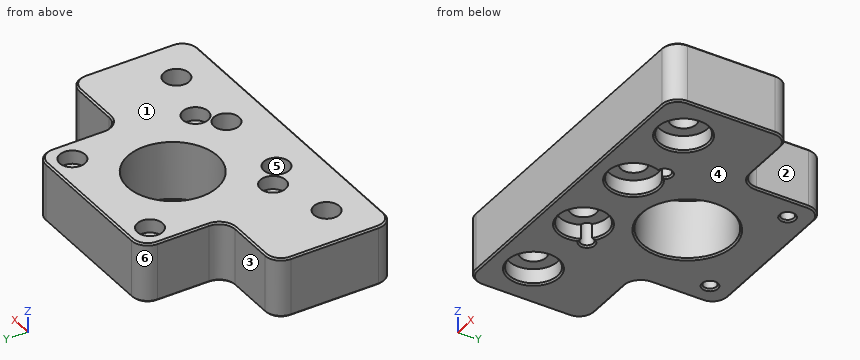
```python
from build123d import *

# Parameters (mm, degrees)
SKETCH_R        = 11.3
SKETCH_R_2      = 1.6
SKETCH_R_3      = 3.2
PAD_DEPTH       = 15
SKETCH001_R     = 3.2
POCKET_DEPTH    = 3.4
SKETCH002_R     = 6.1
POCKET001_DEPTH = 4
FILLET_R        = 4
CHAMFER_SIZE    = 0.4
CHAMFER001_SIZE = 0.4


with BuildPart() as part:
    # Sketch → Pad (new body)
    with BuildSketch(Plane.XY):
        Polygon((20, 30), (20, 51), (62.3, 51), (62.3, 30), (82.3, 30), (82.3, 0), (0, 0), (0, 30), align=None)
        with Locations((41.15, 29.85)):
            Circle(SKETCH_R, mode=Mode.SUBTRACT)
        with Locations((25.65, 45.35)):
            Circle(SKETCH_R_2, mode=Mode.SUBTRACT)
        with Locations((25.65, 14.35)):
            Circle(SKETCH_R_2, mode=Mode.SUBTRACT)
        with Locations((56.65, 45.35)):
            Circle(SKETCH_R_2, mode=Mode.SUBTRACT)
        with Locations((56.65, 14.35)):
            Circle(SKETCH_R_2, mode=Mode.SUBTRACT)
        with Locations((11.15, 10)):
            Circle(SKETCH_R_3, mode=Mode.SUBTRACT)
        with Locations((31.15, 10)):
            Circle(SKETCH_R_3, mode=Mode.SUBTRACT)
        with Locations((51.15, 10)):
            Circle(SKETCH_R_3, mode=Mode.SUBTRACT)
        with Locations((71.15, 10)):
            Circle(SKETCH_R_3, mode=Mode.SUBTRACT)
    extrude(amount=PAD_DEPTH)

    # Sketch001 (on Face19 of Pad) → Pocket (cut)
    with BuildSketch(Plane.XY.offset(15)):
        with Locations((25.65, 45.35)):
            Circle(SKETCH001_R)
        with Locations((56.65, 45.35)):
            Circle(SKETCH001_R)
        with Locations((56.65, 14.35)):
            Circle(SKETCH001_R)
        with Locations((25.65, 14.35)):
            Circle(SKETCH001_R)
    extrude(amount=-POCKET_DEPTH, mode=Mode.SUBTRACT)

    # Sketch002 (on Face4 of Pocket) → Pocket001 (cut)
    with BuildSketch(Plane(origin=(0, 0, 0), x_dir=(1, 0, 0), z_dir=(0, 0, -1))):
        with Locations((11.15, -10)):
            Circle(SKETCH002_R)
        with Locations((31.15, -10)):
            Circle(SKETCH002_R)
        with Locations((51.15, -10)):
            Circle(SKETCH002_R)
        with Locations((71.15, -10)):
            Circle(SKETCH002_R)
    extrude(amount=-POCKET001_DEPTH, mode=Mode.SUBTRACT)

    # Fillet
    fillet_edges = [part.edges().sort_by_distance(p)[0] for p in [
        (62.3, 51, 7.5),
        (62.3, 30, 7.5),
        (82.3, 30, 7.5),
        (82.3, 0, 7.5),
        (0, 0, 7.5),
        (0, 30, 7.5),
        (20, 30, 7.5),
        (20, 51, 7.5),
    ]]
    fillet(fillet_edges, radius=FILLET_R)

    # Chamfer
    chamfer_edges = [part.edges().sort_by_distance(p)[0] for p in [
        (20, 40.5, 0),
        (18.828427, 31.171573, 0),
        (21.171573, 49.828427, 0),
        (10, 30, 0),
        (41.15, 51, 0),
        (1.171573, 28.828427, 0),
        (61.128427, 49.828427, 0),
        (0, 15, 0),
        (62.3, 40.5, 0),
        (1.171573, 1.171573, 0),
        (63.471573, 31.171573, 0),
        (41.15, 0, 0),
        (72.3, 30, 0),
        (81.128427, 1.171573, 0),
        (81.128427, 28.828427, 0),
        (82.3, 15, 0),
        (65.05, 10, 0),
        (57.761563, 13.199162, 0),
        (57.083854, 11.413995, 0),
        (45.618717, 7.428053, 0),
        (56.807929, 15.942187, 0),
        (33.721947, 15.531283, 0),
        (29.736005, 4.066146, 0),
        (24.395064, 15.34254, 0),
        (5.05, 10, 0),
        (55.05, 45.35, 0),
        (29.85, 29.85, 0),
        (24.05, 45.35, 0),
    ]]
    chamfer(chamfer_edges, length=CHAMFER_SIZE)

    # Chamfer001
    chamfer001_edges = [part.edges().sort_by_distance(p)[0] for p in [
        (20, 40.5, 15),
        (21.171573, 49.828427, 15),
        (41.15, 51, 15),
        (61.128427, 49.828427, 15),
        (62.3, 40.5, 15),
        (63.471573, 31.171573, 15),
        (72.3, 30, 15),
        (81.128427, 28.828427, 15),
        (82.3, 15, 15),
        (81.128427, 1.171573, 15),
        (41.15, 0, 15),
        (1.171573, 1.171573, 15),
        (0, 15, 15),
        (1.171573, 28.828427, 15),
        (10, 30, 15),
        (18.828427, 31.171573, 15),
    ]]
    chamfer(chamfer001_edges, length=CHAMFER001_SIZE)


solid = part.part
```
CAD build for the part. Positions are in the model's coordinates, mm. Face numbers are marked on the shaded views. A direction names the side the tool comes from. Round coordinates to 2 decimals unless told otherwise and drop trailing zeros. Write each loop counter-clockwise with the first axis right and the second up, starting at its lowest first coordinate (ties: lowest second). Pieces come first, ordered by that corner, then holes. Notation, with made-up numbers: (21, 88.5) - (70, 88.5) arc R34 cw to (70, 120.5) - close; hole circle Ø1 at (26, 29.25). An arc over 180 degrees is marked (long way). Write item = value, one per line. Start each with the question number.
Q1. Probe L1, parallel to X at y = 10, z = 8; L2, parallel to Y at x = 56.65, z = 4.5; L3, parallel to X at y = 10, z = 2.1. List the from-to ranges inside material, lowest first. Write a range as from..to.
Q2. Mould opens along X. For the marked faces 4, 5 and 6 say: pulls with the +X half, pulls with the -X half, needs draft (parallel to the pull), parting line crosses it, or undercut.
Q3. Which spindle directions (+Z, -Z, +X, -X, +Y, -Y) get a long thin tool onto all of the face, cutting with end or side? Do the marked faces 1, 2 and 3. Say none if no direction does.
Q4. Drop flat-ended pins along their axis: pin 1 (7 mm diameter, centred on x = 26.5, y = 45, fed in from +Z); pin 2 (6.5 mm diameter, centred on y = 42.5, z = 6.5, fed in from -X); pin 3 (1.9 mm diameter, centred on x = 57, y = 47, fed in from +Z); pin 4 (3 mm diameter, centred on x = 72, z = 12.5, fed in from +Y). Give the stop position or say it passes through.
Q5. Band-saw the part on B-B (z = 12.75). Count the separate pieces of the cut face and the enclosed holes in it, then the cut area to 3 significant figures.
Q6. Band-saw the part on A-A (x = 41.15). Give the cut face in (y, z), then the cut area to 3 significant figures.
Answers below:
q1.L1 = 0..7.95, 14.35..27.95, 34.35..47.95, 54.35..67.95, 74.35..82.3
q1.L2 = 0..12.75, 15.95..43.75, 46.95..51
q1.L3 = 0..5.05, 17.25..25.05, 37.25..45.05, 57.25..65.05, 77.25..82.3
q2.face_4 = needs draft
q2.face_5 = undercut
q2.face_6 = pulls with the -X half
q3.face_1 = +Z, +X, -X, +Y, -Y
q3.face_2 = +Z, -Z, +X, +Y
q3.face_3 = +Z, -Z, -X, +Y
q4.pin_1 = 15
q4.pin_2 = 20
q4.pin_3 = 11.6
q4.pin_4 = 30
q5.separate_pieces = 1
q5.enclosed_holes = 9
q5.area = 2,690 mm2
q6.outline = (0, 0.4) - (0.4, 0) - (18.15, 0) - (18.55, 0.4) - (18.55, 15) - (0.4, 15) - (0, 14.6) - close; (41.15, 0.4) - (41.55, 0) - (50.6, 0) - (51, 0.4) - (51, 14.6) - (50.6, 15) - (41.15, 15) - close
q6.area = 426 mm2
